Part print with two shaded views. Sizes in mm from the minimum x, y, z corner. A direction names the side the tool comes from. Coordinates: 2 decimals unless noted, no trailing zeros. Loops run counter-clockwise (first coordinate to the right, second up) from the corner with the lowest first, then second, coordinate; pieces in that order, holes last.
(1) Wall check: L1, parallel to Y at x = 3, z = 0.9; L2, parallel to Z at x = 4, y = 47.5; L3, parallel to Z at x = 2.5, y = 7. Give the ranges that are in metal, low to high.
(2) Slice it at B-B (y = 24). Give the cut face in (x, z).
(3) Slice it at A-A (x = 3). Give the cut face in (y, z), and give its area (3 significant figures).
(4) Slice it at D-D (z = 5). Give the cut face in (x, y).
(5) Tool access for the marked faces 1, 2 and 3: list every direction of +Z, -Z, +X, -X, +Y, -Y with a clear straight run to the whole face (end or side of a thin tool).
(6) Slice it at C-C (z = 0.75). Give the cut face in (x, y).
(7) Flat gauge pins, fed straight in: P1, Ø1.8, axis at x = 1.5, z = 4, coming from the -Y side; P2, Ø2, axis at x = 4, y = 1.5, coming from the +Z side. Where does each tip first touch, or does it go through?
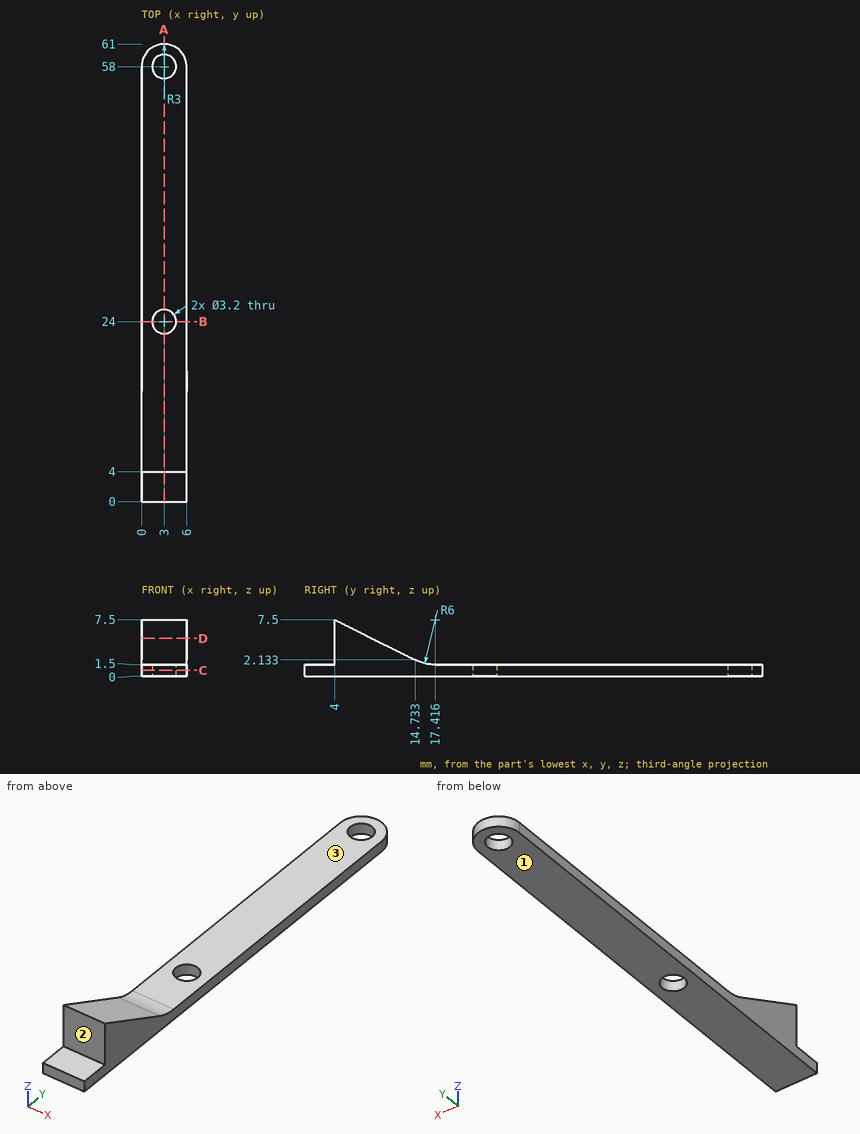
Response values:
1. L1: y = 0 to 22.4, 25.6 to 56.4, 59.6 to 61
1. L2: z = 0 to 1.5
1. L3: z = 0 to 6
2. outline: (0, 0) - (1.4, 0) - (1.4, 1.5) - (0, 1.5) - close; (4.6, 0) - (6, 0) - (6, 1.5) - (4.6, 1.5) - close
3. outline: (0, 0) - (22.4, 0) - (22.4, 1.5) - (17.42, 1.5) arc R6 cw to (14.73, 2.13) - (4, 7.5) - (4, 1.5) - (0, 1.5) - close; (25.6, 0) - (56.4, 0) - (56.4, 1.5) - (25.6, 1.5) - close; (59.6, 0) - (61, 0) - (61, 1.5) - (59.6, 1.5) - close
3. area: 118 mm2
4. outline: (0, 4) - (6, 4) - (6, 9) - (0, 9) - close
5. face 1: -Z, +X, -X, +Y, -Y
5. face 2: +Z, +X, -X, -Y
5. face 3: +Z, +X, -X, +Y
6. outline: (0, 0) - (6, 0) - (6, 58) arc R3 ccw to (0, 58) - close; hole circle Ø3.2 at (3, 24); hole circle Ø3.2 at (3, 58)
7. P1: stops at y = 4
7. P2: stops at z = 1.5
